```python
from build123d import *

# Parameters (mm, degrees)
SKETCH1_W               = 51.961524228
SKETCH1_H               = 30
SKETCH1_R               = 5
BOSS_EXTRUDE1_DEPTH     = 14.5
SKETCH2_W               = 29
SKETCH2_H               = 51.961524228
BOSS_EXTRUDE2_DEPTH     = 15
SKETCH3_W               = 72
SKETCH3_H               = 125
SKETCH3_R               = 5
BOSS_EXTRUDE3_DEPTH     = 10
FILLET1_R               = 20
CUT_EXTRUDE1_DEPTH      = 83.475754013
CUT_EXTRUDE1_DEPTH_BACK = 83.475754013
SKETCH4_R               = 5
CUT_EXTRUDE2_DEPTH      = 137.091880728
CUT_EXTRUDE2_DEPTH_BACK = 137.091880728
SKETCH5_W               = 42
SKETCH5_H               = 6
CUT_EXTRUDE3_DEPTH      = 104.393665183
CUT_EXTRUDE3_DEPTH_BACK = 104.393665183
SKETCH6_R               = 2.5


with BuildPart() as part:
    # Sketch1 → Boss-Extrude1 (new, symmetric)
    with BuildSketch(Plane(origin=(0, 0, 0), x_dir=(0, 0, -1), z_dir=(1, 0, 0))):
        Rectangle(SKETCH1_W, SKETCH1_H)
        with Locations(Location((0, 0, 0), (0, 0, 180))):
            Circle(SKETCH1_R, mode=Mode.SUBTRACT)
    extrude(amount=BOSS_EXTRUDE1_DEPTH, both=True)

    # Sketch2 → Boss-Extrude2 (add)
    with BuildSketch(Plane(origin=(0, 15, 0), x_dir=(1, 0, 0), z_dir=(0, 1, 0))):
        Rectangle(SKETCH2_W, SKETCH2_H)
    extrude(amount=BOSS_EXTRUDE2_DEPTH)

    # Sketch3 → Boss-Extrude3 (add)
    with BuildSketch(Plane(origin=(0, 30, 0), x_dir=(1, 0, 0), z_dir=(0, 1, 0))):
        Rectangle(SKETCH3_W, SKETCH3_H)
        with Locations(Location((-27.36, 47.5, 0), (0, 0, 270))):
            Circle(SKETCH3_R, mode=Mode.SUBTRACT)
        with Locations(Location((27.36, 47.5, 0), (0, 0, 270))):
            Circle(SKETCH3_R, mode=Mode.SUBTRACT)
        with Locations(Location((-27.36, -47.5, 0), (0, 0, 270))):
            Circle(SKETCH3_R, mode=Mode.SUBTRACT)
        with Locations(Location((27.36, -47.5, 0), (0, 0, 270))):
            Circle(SKETCH3_R, mode=Mode.SUBTRACT)
    extrude(amount=BOSS_EXTRUDE3_DEPTH)

    # Fillet1
    fillet1_edges = [part.edges().sort_by_distance(p)[0] for p in [
        (0, -15, 25.980762114),
        (0, -15, -25.980762114),
    ]]
    fillet(fillet1_edges, radius=FILLET1_R)

    # Sketch4 → Cut-Extrude1 (cut, two sides: drawn at the far end of the back side and taken through both)
    with BuildSketch(Plane.XY.offset(-CUT_EXTRUDE1_DEPTH_BACK)):
        with Locations(Location((0, 0, 0), (0, 0, 90))):
            Circle(SKETCH4_R)
    extrude(amount=CUT_EXTRUDE1_DEPTH + CUT_EXTRUDE1_DEPTH_BACK, mode=Mode.SUBTRACT)

    # Sketch5 → Cut-Extrude2 (cut, two sides: drawn at the far end of the back side and taken through both)
    with BuildSketch(Plane.XY.offset(62.5).offset(-CUT_EXTRUDE2_DEPTH_BACK)):
        with Locations((0, 37)):
            Rectangle(SKETCH5_W, SKETCH5_H)
    extrude(amount=CUT_EXTRUDE2_DEPTH + CUT_EXTRUDE2_DEPTH_BACK, mode=Mode.SUBTRACT)

    # Sketch6 → Cut-Extrude3 (cut, two sides: drawn at the far end of the back side and taken through both)
    with BuildSketch(Plane(origin=(36, 0, 0), x_dir=(0, 0, -1), z_dir=(1, 0, 0)).offset(-CUT_EXTRUDE3_DEPTH_BACK)):
        with Locations((-25, 35)):
            Circle(SKETCH6_R)
        with Locations((25, 35)):
            Circle(SKETCH6_R)
    extrude(amount=CUT_EXTRUDE3_DEPTH + CUT_EXTRUDE3_DEPTH_BACK, mode=Mode.SUBTRACT)


solid = part.part
```
Source: CAD feature listing. Evaluate the final solid. Frame: model axes, mm. A direction names the side the tool comes from. Give positions to 0.01 mm unless a question says otherwise; leave off trailing zeros. Loops run counter-clockwise (first coordinate to the right, second up) from the corner with the lowest first, then second, coordinate; pieces in that order, holes last. Notation, with made-up numbers: (38.25, 21) -> (80.25, 21) arc R29 cw to (80.25, 60) -> close; hole circle Ø7 at (-36, 70). An arc over 180 degrees is marked (long way). Put each result on its own line as item: value. Start each with the question number.
1) Cut plane D-D (y = 0). Return loops of the section in (x, z).
2) Material intervals for probe 1 along X at (y, z) = (35.5, -47.5); probe 2 along Y at (x, z) = (6, 0); probe 3 along Y at (x, z) = (28, -16), sorted ascending.
3) Reachability of faces 5 (the face through (0, 17, 25.981)), 6 (the face through (-14.5, 7, 0)), 7 (the face through (0, 34, 45)), 8 (the face through (14.5, 7, 0)) from +Z, -Z, +X, -X, +Y, -Y: full face, straight path, thin tool, end or side. Return the list, or none.
4) Cut plane C-C (x = -27.36). Return loops of the section in (y, z).
5) Cut plane B-B (z = -47.5). Return loops of the section in (x, y), then the cut area to 3 significant figures.
6) Contact query for flat-ended pins moving along their axis: P1, Ø5, axis at x = 4.5, y = 1, coming from the +Z side; P2, Ø10.5, axis at x = -8, z = 42.5, coming from the +Y side; P3, Ø11.5, axis at x = 0, y = 0, coming from the -Z side. Output: stop coordinate, or through.
7) Cut plane A-A (x = -12.5). Return loops of the section in (y, z).
8) Draft query along Z for faces 1 (the face through (24.32, 34.93, 43.53)), 2 (the face through (0, 34, -45)), 3 (the face through (0.203, -8.986, -20.278)), 4 (the face through (0.203, -8.986, 20.278)). Return one class per face: released by +Z, released by -Z, zero draft, split by the parting line, or undercut.
Results are:
1. outline: (-14.5, -25.35) -> (-5, -25.35) -> (-5, -5) -> (-14.5, -5) -> close; (-14.5, 5) -> (-5, 5) -> (-5, 25.35) -> (-14.5, 25.35) -> close; (5, -25.35) -> (14.5, -25.35) -> (14.5, -5) -> (5, -5) -> close; (5, 5) -> (14.5, 5) -> (14.5, 25.35) -> (5, 25.35) -> close
2. probe 1: x = -36 to -32.36, -22.36 to -21, 21 to 22.36, 32.36 to 36
2. probe 2: y = -15 to -5, 5 to 34
2. probe 3: y = 30 to 40
3. face 5: +Z, +X, -X, -Y
3. face 6: +Z, -Z, -X, -Y
3. face 7: +Z, -Z, +Y
3. face 8: +Z, -Z, +X, -Y
4. outline: (30, -62.5) -> (40, -62.5) -> (40, -52.5) -> (30, -52.5) -> close; (30, -42.5) -> (40, -42.5) -> (40, 42.5) -> (30, 42.5) -> close; (30, 52.5) -> (40, 52.5) -> (40, 62.5) -> (30, 62.5) -> close; hole circle Ø5 at (35, -25); hole circle Ø5 at (35, 25)
5. outline: (-36, 30) -> (-32.36, 30) -> (-32.36, 40) -> (-36, 40) -> close; (-22.36, 30) -> (22.36, 30) -> (22.36, 40) -> (21, 40) -> (21, 34) -> (-21, 34) -> (-21, 40) -> (-22.36, 40) -> close; (32.36, 30) -> (36, 30) -> (36, 40) -> (32.36, 40) -> close
5. area: 268 mm2
6. P1: stops at z = 25.92
6. P2: stops at y = 34
6. P3: stops at z = -25.98
7. outline: (-15, -5.98) arc R20 ccw to (5, -25.98) -> (30, -25.98) -> (30, -62.5) -> (34, -62.5) -> (34, -27.29) arc R2.5 cw to (34, -22.71) -> (34, 22.71) arc R2.5 cw to (34, 27.29) -> (34, 62.5) -> (30, 62.5) -> (30, 25.98) -> (5, 25.98) arc R20 ccw to (-15, 5.98) -> close; hole circle Ø10 at (0, 0)
8. face 1: undercut
8. face 2: zero draft
8. face 3: released by -Z
8. face 4: released by +Z
